```python
from build123d import *

# Parameters (mm, degrees)
SKETCH1_W           = 112.776
SKETCH1_H           = 96.774
BOSS_EXTRUDE1_DEPTH = 25.4
SKETCH2_R           = 8.334375
CUT_EXTRUDE2_DEPTH  = 151.760715215
SKETCH3_R           = 8.334375
CUT_EXTRUDE4_DEPTH  = 151.760715215
SKETCH4_R           = 3.571875
CUT_EXTRUDE6_DEPTH  = 7.874
SKETCH5_R           = 3.571875
CUT_EXTRUDE8_DEPTH  = 7.874
CUT_EXTRUDE10_START = 25.4
SKETCH6_R           = 3.175
CUT_EXTRUDE10_DEPTH = 7.874
CUT_EXTRUDE12_START = 25.4
SKETCH7_R           = 3.175
CUT_EXTRUDE12_DEPTH = 7.874
CUT_EXTRUDE14_START = 25.4
SKETCH8_R           = 16.6497
CUT_EXTRUDE14_DEPTH = 2.8194
CUT_EXTRUDE15_START = 25.4
SKETCH9_R           = 16.6497
CUT_EXTRUDE15_DEPTH = 2.8194


with BuildPart() as part:
    # Sketch1 → Boss-Extrude1 (new body)
    with BuildSketch(Plane.YZ):
        with Locations((56.388, 48.387)):
            Rectangle(SKETCH1_W, SKETCH1_H)
    extrude(amount=BOSS_EXTRUDE1_DEPTH)

    # Sketch2 → Cut-Extrude2 (cut, through all)
    with BuildSketch(Plane.YZ):
        with Locations(Location((15.875, 15.875, 0), (0, 0, 270))):
            Circle(SKETCH2_R)
    extrude(amount=CUT_EXTRUDE2_DEPTH, mode=Mode.SUBTRACT)

    # Sketch3 → Cut-Extrude4 (cut, through all)
    with BuildSketch(Plane.YZ):
        with Locations(Location((96.901, 15.875, 0), (0, 0, 270))):
            Circle(SKETCH3_R)
        with Locations(Location((15.875, 80.899, 0), (0, 0, 270))):
            Circle(SKETCH3_R)
        with Locations(Location((96.901, 80.899, 0), (0, 0, 270))):
            Circle(SKETCH3_R)
    extrude(amount=CUT_EXTRUDE4_DEPTH, mode=Mode.SUBTRACT)

    # Sketch4 → Cut-Extrude6 (cut)
    with BuildSketch(Plane.YZ):
        with Locations(Location((105.537, 48.387, 0), (0, 0, 270))):
            Circle(SKETCH4_R)
    extrude(amount=CUT_EXTRUDE6_DEPTH, mode=Mode.SUBTRACT)

    # Sketch5 → Cut-Extrude8 (cut)
    with BuildSketch(Plane.YZ):
        with Locations(Location((56.515, 15.875, 0), (0, 0, 270))):
            Circle(SKETCH5_R)
    extrude(amount=CUT_EXTRUDE8_DEPTH, mode=Mode.SUBTRACT)

    # Sketch6 → Cut-Extrude10 (cut)
    with BuildSketch(Plane.YZ.offset(CUT_EXTRUDE10_START)):
        with Locations(Location((7.239, 48.387, 0), (0, 0, 270))):
            Circle(SKETCH6_R)
    extrude(amount=-CUT_EXTRUDE10_DEPTH, mode=Mode.SUBTRACT)

    # Sketch7 → Cut-Extrude12 (cut)
    with BuildSketch(Plane.YZ.offset(CUT_EXTRUDE12_START)):
        with Locations(Location((56.261, 80.899, 0), (0, 0, 270))):
            Circle(SKETCH7_R)
    extrude(amount=-CUT_EXTRUDE12_DEPTH, mode=Mode.SUBTRACT)

    # Sketch8 → Cut-Extrude14 (cut)
    with BuildSketch(Plane.YZ.offset(CUT_EXTRUDE14_START)):
        with Locations(Location((38.227, 48.387, 0), (0, 0, 270))):
            Circle(SKETCH8_R)
    extrude(amount=-CUT_EXTRUDE14_DEPTH, mode=Mode.SUBTRACT)

    # Sketch9 → Cut-Extrude15 (cut)
    with BuildSketch(Plane.YZ.offset(CUT_EXTRUDE15_START)):
        with Locations(Location((84.201, 48.387, 0), (0, 0, 270))):
            Circle(SKETCH9_R)
    extrude(amount=-CUT_EXTRUDE15_DEPTH, mode=Mode.SUBTRACT)


solid = part.part
```
The listing builds one solid part. Answer for the finished solid, in the listing's coordinates (mm). A direction names the side the tool comes from. Coordinates: 2 decimals unless noted, no trailing zeros. Loops run counter-clockwise (first coordinate to the right, second up) from the corner with the lowest first, then second, coordinate; pieces in that order, holes last. Notation, with made-up numbers: (3, 60) - (27, 60) arc R28 cw to (27, 91) - close; hole circle Ø10 at (87, 80). An arc over 180 degrees is marked (long way). Write item = value, one per line.
1) Which of the six approach directions +Z, -Z, +X, -X, +Y, -Y give full straight-line access (tool end or side, diameter ignored) to faces 1 (the face through (12.52, 16.24, 24.2)), 2 (the face through (7.874, 106, 48)), 3 (the face through (22.581, 38, 49))?
Responses:
face_1 = +X, -X
face_2 = -X
face_3 = +X
2) Determine the mould class of faces 4 (the face through (0, 56, 49)), 5 (the face through (13, 0, 48)), 6 (the face through (24.01, 89.202, 32.506)), 7 (the face through (21.52, 54.33, 83.42)) for opening direction Y: pulls with the +Y half, pulls with the -Y half, needs draft (parallel to the pull), parting line crosses it, or undercut.
Responses:
face_4 = needs draft
face_5 = pulls with the -Y half
face_6 = undercut
face_7 = undercut
3) Section B-B (z = 11) is taken. Determine the outline of the cut face in (x, y), plus the area to 3 significant figures.
Responses:
outline = (0, 0) - (25.4, 0) - (25.4, 9.12) - (0, 9.12) - close; (0, 22.63) - (25.4, 22.63) - (25.4, 90.14) - (0, 90.14) - close; (0, 103.66) - (25.4, 103.66) - (25.4, 112.78) - (0, 112.78) - close
area = 2,180 mm^2
4) Find the intervals of material crossed by line 1 along Y through (x, z) = (18.5, 76); line 2 along Y through (x, z) = (24.25, 34.5); line 3 along Z through (x, y) = (13.75, 94), in increasing order.
Responses:
line_1 = 0 to 9.13, 22.62 to 90.16, 103.64 to 112.78
line_2 = 0 to 29.04, 47.41 to 75.02, 93.39 to 112.78
line_3 = 0 to 8.06, 23.69 to 73.09, 88.71 to 96.77
5) Section D-D (z = 42.5) is taken. Determine the outline of the cut face in (x, y), plus the area to 3 significant figures.
Responses:
outline = (0, 0) - (25.4, 0) - (25.4, 22.65) - (22.58, 22.65) - (22.58, 53.8) - (25.4, 53.8) - (25.4, 68.63) - (22.58, 68.63) - (22.58, 99.78) - (25.4, 99.78) - (25.4, 112.78) - (0, 112.78) - close
area = 2,690 mm^2
6) Section C-C (y = 28) is taken. Determine the outline of the cut face in (x, z), plus the area to 3 significant figures.
Responses:
outline = (0, 0) - (25.4, 0) - (25.4, 35.25) - (22.58, 35.25) - (22.58, 61.53) - (25.4, 61.53) - (25.4, 96.77) - (0, 96.77) - close
area = 2,380 mm^2
7) Each of these flat-tipped pins is pushed along its axis until it touches: P1, Ø1.9, axis at y = 6.5, z = 48.5, coming from the +X side; P2, Ø10, axis at y = 96.901, z = 80.899, coming from the +X side; P3, Ø5, axis at y = 75, z = 41.5, coming from the +X side; P4, Ø3.5, axis at y = 104, z = 48, coming from the -X side. Where does it stop, or does it pass through?
Responses:
P1 = 17.53
P2 = through
P3 = 22.58
P4 = 7.87
8) Section A-A (x = 19.75) is taken. Determine the outline of the cut face in (y, z) (3 decimals), plus the area to 3 significant figures.
Responses:
outline = (0, 0) - (112.776, 0) - (112.776, 96.774) - (0, 96.774) - close; hole circle Ø6.35 at (7.239, 48.387); hole circle Ø16.669 at (15.875, 15.875); hole circle Ø16.669 at (15.875, 80.899); hole circle Ø6.35 at (56.261, 80.899); hole circle Ø16.669 at (96.901, 15.875); hole circle Ø16.669 at (96.901, 80.899)
area = 9,980 mm^2
